The model under review builds one solid part; all positions refer to its coordinate system, in mm. A direction names the side the tool comes from. Round coordinates to 2 decimals unless told otherwise and drop trailing zeros. Put each result on its own line as item: value. Start each with the question number.
from build123d import *

# Parameters (mm, degrees)
PAD004_DEPTH        = 3
POCKET007_DEPTH     = 3.001
POCKET008_DEPTH     = 3.001
POCKET009_DEPTH     = 3.001
POCKET010_DEPTH     = 3.001
POCKET011_DEPTH     = 3.001
POCKET012_DEPTH     = 3.001
POCKET013_DEPTH     = 3.001
POCKET014_DEPTH     = 3.001
POCKET015_DEPTH     = 3.001
COPYCOPYSKETCH023_R = 3.5
POCKET033_DEPTH     = 5


with BuildPart() as part:
    # Sketch012 → Pad004 (new body)
    with BuildSketch(Plane.XY):
        with BuildLine():
            Line((0, 67.42), (0, -55.65))
            Line((0, -55.65), (-117.94, -55.65))
            ThreePointArc((-127.64, -49.11), (-122.947197, -52.613151), (-117.94, -55.65))
            ThreePointArc((-146.95, -26.77), (-138.520798, -38.999541), (-127.64, -49.11))
            ThreePointArc((-148.54, 6.09), (-150.980867, -10.496574), (-146.95, -26.77))
            ThreePointArc((-134.5, 26.2), (-142.831473, 17.060618), (-148.54, 6.09))
            ThreePointArc((-94.13, 48.54), (-115.023795, 38.650843), (-134.5, 26.2))
            ThreePointArc((0, 67.42), (-48.036997, 62.826084), (-94.13, 48.54))
        make_face()
    extrude(amount=PAD004_DEPTH)

    # CopySketch001 → Pocket007 (cut, through all)
    with BuildSketch(Plane.XY.offset(3)):
        with BuildLine():
            ThreePointArc((0, 22), (-24.535688, 7.490738), (-23.643181, -21))
            Line((-23.643181, -21), (0, -21))
            Line((0, -21), (0, 22))
        make_face()
        with BuildLine():
            ThreePointArc((-45.15951, 13.5), (-47.417918, 19.740491), (-53.752095, 17.76))
            ThreePointArc((-53.752095, 17.76), (-58.626578, 4.267932), (-60.018385, -10.01))
            ThreePointArc((-60.018385, -10.01), (-55.15457, -14.259051), (-50.463519, -9.82))
            ThreePointArc((-45.15951, 13.5), (-49.299707, 2.178481), (-50.463519, -9.82))
        make_face()
    extrude(amount=-POCKET007_DEPTH, mode=Mode.SUBTRACT)

    # CopySketch002 → Pocket008 (cut, through all)
    with BuildSketch(Plane.XY.offset(3)):
        with BuildLine():
            ThreePointArc((-49.444058, -22.5277), (-54.944649, -19.654794), (-58.184448, -24.9476))
            Line((-57.0427, -29.8572), (-58.184448, -24.9476))
            ThreePointArc((-60.1254, -35.4518), (-57.027903, -33.511958), (-57.0427, -29.8572))
            ThreePointArc((-80.4488, -36.935), (-70.225534, -37.037002), (-60.1254, -35.4518))
            Line((-97.9175, -34.995), (-80.4488, -36.935))
            ThreePointArc((-97.9175, -34.995), (-103.82056, -38.432829), (-99.6413, -43.8364))
            ThreePointArc((-99.6413, -43.8364), (-82.042265, -45.74625), (-64.34, -45.6882))
            ThreePointArc((-64.34, -45.6882), (-56.228822, -44.011588), (-48.7903, -40.3687))
            ThreePointArc((-48.7903, -40.3687), (-46.155403, -37.339305), (-45.3966, -33.3967))
            Line((-49.444058, -22.5277), (-45.3966, -33.3967))
        make_face()
    extrude(amount=-POCKET008_DEPTH, mode=Mode.SUBTRACT)

    # CopySketch003 → Pocket009 (cut, through all)
    with BuildSketch(Plane.XY.offset(3)):
        with BuildLine():
            ThreePointArc((-64.365395, -8.62779), (-67.742586, -5.639295), (-70.674058, -9.0661))
            ThreePointArc((-70.674058, -9.0661), (-70.835475, -15.903269), (-70.2223, -22.7148))
            ThreePointArc((-71.4121, -25.164), (-70.40839, -24.137996), (-70.2223, -22.7148))
            ThreePointArc((-87.147068, -25.4704), (-79.265214, -26.055148), (-71.4121, -25.164))
            ThreePointArc((-87.147068, -25.4704), (-90.683175, -28.650592), (-87.411994, -32.1027))
            ThreePointArc((-87.411994, -32.1027), (-76.595145, -33.065808), (-65.7651, -32.2646))
            ThreePointArc((-65.7651, -32.2646), (-63.346864, -30.693689), (-62.8224, -27.8581))
            ThreePointArc((-64.365395, -8.62779), (-64.044087, -18.279067), (-62.8224, -27.8581))
        make_face()
    extrude(amount=-POCKET009_DEPTH, mode=Mode.SUBTRACT)

    # CopySketch018 → Pocket010 (cut, through all)
    with BuildSketch(Plane.XY.offset(3)):
        with BuildLine():
            ThreePointArc((-72.02, 14.094017), (-72.392692, 16.846151), (-74.97, 17.880861))
            ThreePointArc((-74.97, 17.880861), (-93.250673, 11.950737), (-109.81, 2.196863))
            ThreePointArc((-109.81, 2.196863), (-114.369998, -5.844169), (-109.82, -13.890864))
            ThreePointArc((-109.82, -13.890864), (-95.344007, -19.39947), (-80, -21.511475))
            ThreePointArc((-80, -21.511475), (-76.570681, -20.127404), (-75.5, -16.587696))
            ThreePointArc((-72.02, 14.094017), (-75.072637, -1.097957), (-75.5, -16.587696))
        make_face()
    extrude(amount=-POCKET010_DEPTH, mode=Mode.SUBTRACT)

    # CopySketch019 → Pocket011 (cut, through all)
    with BuildSketch(Plane.XY.offset(3)):
        with BuildLine():
            ThreePointArc((-98.800419, -30.00485), (-94.734065, -27.856904), (-96.886613, -23.792983))
            ThreePointArc((-116.257935, -13.543183), (-107.162558, -19.783674), (-96.886613, -23.792983))
            ThreePointArc((-115.288548, 4.68), (-118.878907, -4.266385), (-116.257935, -13.543183))
            ThreePointArc((-115.288548, 4.68), (-115.784536, 8.891716), (-120.0081, 8.509533))
            ThreePointArc((-120.0081, 8.509533), (-126.190374, -3.981903), (-122.223343, -17.343009))
            ThreePointArc((-122.223343, -17.343009), (-111.413274, -25.3414), (-98.800419, -30.00485))
        make_face()
    extrude(amount=-POCKET011_DEPTH, mode=Mode.SUBTRACT)

    # CopySketch020 → Pocket012 (cut, through all)
    with BuildSketch(Plane.XY.offset(3)):
        with BuildLine():
            ThreePointArc((-103.601499, 24.683247), (-102.23683, 28.460376), (-105.872604, 30.166298))
            ThreePointArc((-105.872604, 30.166298), (-120.215401, 22.727476), (-132.072524, 11.752025))
            ThreePointArc((-132.072524, 11.752025), (-139.729925, -7.755401), (-131.983106, -27.22749))
            ThreePointArc((-131.983106, -27.22749), (-123.229381, -34.095551), (-113.177794, -38.866668))
            ThreePointArc((-113.177794, -38.866668), (-108.540165, -37.030837), (-109.968182, -32.251858))
            ThreePointArc((-126.694192, -19.799013), (-118.971743, -26.885797), (-109.968182, -32.251858))
            ThreePointArc((-126.624592, 8.183725), (-131.669932, -5.795181), (-126.694192, -19.799013))
            ThreePointArc((-103.601499, 24.683247), (-116.290857, 18.07698), (-126.624592, 8.183725))
        make_face()
    extrude(amount=-POCKET012_DEPTH, mode=Mode.SUBTRACT)

    # CopySketch021 → Pocket013 (cut, through all)
    with BuildSketch(Plane.XY.offset(3)):
        with BuildLine():
            ThreePointArc((-50.283742, 31.504046), (-49.647546, 34.54879), (-52.191507, 36.338616))
            ThreePointArc((-52.191507, 36.338616), (-81.328643, 28.362539), (-109.1608, 16.616836))
            ThreePointArc((-109.1608, 16.616836), (-110.288036, 12.383863), (-106.13456, 10.991977))
            ThreePointArc((-64.402467, 26.573807), (-85.690853, 19.914024), (-106.13456, 10.991977))
            ThreePointArc((-62.78, 24.679977), (-62.809905, 26.296266), (-64.402467, 26.573807))
            ThreePointArc((-62.78, 24.679977), (-67.226683, 14.561044), (-69.887292, 3.833184))
            ThreePointArc((-69.887292, 3.833184), (-67.736073, 0.176429), (-64.257156, 2.604748))
            ThreePointArc((-50.283742, 31.504046), (-59.288565, 18.030198), (-64.257156, 2.604748))
        make_face()
    extrude(amount=-POCKET013_DEPTH, mode=Mode.SUBTRACT)

    # CopySketch021001 → Pocket014 (cut, through all)
    with BuildSketch(Plane.XY.offset(3)):
        with BuildLine():
            ThreePointArc((-50.283742, 31.504046), (-49.647546, 34.54879), (-52.191507, 36.338616))
            ThreePointArc((-52.191507, 36.338616), (-81.328643, 28.362539), (-109.1608, 16.616836))
            ThreePointArc((-109.1608, 16.616836), (-110.288036, 12.383863), (-106.13456, 10.991977))
            ThreePointArc((-64.402467, 26.573807), (-85.690853, 19.914024), (-106.13456, 10.991977))
            ThreePointArc((-62.78, 24.679977), (-62.809905, 26.296266), (-64.402467, 26.573807))
            ThreePointArc((-62.78, 24.679977), (-67.226683, 14.561044), (-69.887292, 3.833184))
            ThreePointArc((-69.887292, 3.833184), (-67.736073, 0.176429), (-64.257156, 2.604748))
            ThreePointArc((-50.283742, 31.504046), (-59.288565, 18.030198), (-64.257156, 2.604748))
        make_face()
    extrude(amount=-POCKET014_DEPTH, mode=Mode.SUBTRACT)

    # CopySketch022 → Pocket015 (cut, through all)
    with BuildSketch(Plane.XY.offset(3)):
        with BuildLine():
            ThreePointArc((-95.442672, 36.502192), (-97.482535, 31.79948), (-92.84279, 29.620188))
            ThreePointArc((-41.465962, 43.393869), (-67.471527, 37.690024), (-92.84279, 29.620188))
            ThreePointArc((-31.493419, 44.517429), (-36.50836, 44.210116), (-41.465962, 43.393869))
            ThreePointArc((-31.299124, 42.370301), (-30.554517, 43.520036), (-31.493419, 44.517429))
            ThreePointArc((-31.299124, 42.370301), (-33.877911, 40.536126), (-36.077509, 38.26102))
            ThreePointArc((-36.077509, 38.26102), (-36.412838, 32.470844), (-30.619491, 32.195671))
            ThreePointArc((-9.425793, 43.552177), (-20.673272, 39.08814), (-30.619491, 32.195671))
            ThreePointArc((-9.425793, 43.552177), (-6.127962, 50.951278), (-12.675069, 55.721791))
            ThreePointArc((-12.675069, 55.721791), (-55.094244, 50.570744), (-95.442672, 36.502192))
        make_face()
    extrude(amount=-POCKET015_DEPTH, mode=Mode.SUBTRACT)

    # CopyCopySketch023 → Pocket033 (cut)
    with BuildSketch(Plane.XY.offset(3)):
        with Locations((-30, -40)):
            Circle(COPYCOPYSKETCH023_R)
    extrude(amount=-POCKET033_DEPTH, mode=Mode.SUBTRACT)


with BuildPart() as part_1:
    # Body003 placement: moved
    add(part.part.moved(Location((0, 0, 83))))


solid = part_1.part
Q1. For faces 1 (the face through (-57.606, -27.437, 84.521)), 2 (the face through (-74, -7, 86)), list the 3-axis set-ups (+Z, -Z, +X, -X, +Y, -Y) from which the entire face can be reached by the end or side of a thin tool; tool diameter is ignored.
Q2. Take a section at A-A on z = 84.15. State how many separate pieces and enclosed holes the cut face has, and give its area (3 significant figures).
Q3. Wall thickness on probe 1 along Y at (x, z) = (-52, 83.65); probe 2 along Y at (x, z) = (-30, 84.65); probe 3 along Y at (x, z) = (-8, 85.85): over which ranges is each line inside the solid? List them lowest first. Write a range as [from, to].
Q4. Draft analysis for pull direction Y (two halves, no side actions). For faces 3 (the face through (0, -38, 84)), 4 (the face through (-150.99, -10.26, 84.48)), 5 (the face through (-79.376, -26.057, 84.521)), state which applies: +Y half, -Y half, draft (parallel to the pull), parting line (faces both ways), or undercut.
Q5. Clearance check with flat-ended pins moving along their axes: pin 1 Ø1.5 at (x, y) = (-77, -9.5) entering from +Z; pin 2 Ø8 at (x, y) = (-30, -40) entering from +Z. State where each tip first meets the part, or that it passes through.
Calculated:
1. face 1: +Z, -Z
1. face 2: +Z, +X, -X, +Y, -Y
2. separate pieces: 1
2. enclosed holes: 9
2. area: 9,330 mm²
3. probe 1: y = [-55.65, -42.23], [-19.83, -12.99], [19.57, 29.49], [36.33, 41.39], [51.26, 62]
3. probe 2: y = [-55.65, -43.5], [-36.5, 32.73], [54.73, 65.72]
3. probe 3: y = [-55.65, -21], [20.83, 44.54], [54.04, 67.34]
4. face 3: draft
4. face 4: parting line
4. face 5: undercut
5. pin 1: passes through
5. pin 2: stops at z = 86
